Design review of the part built by this model. Coordinates are the model's own, in mm. Face numbers are marked on the shaded views. Coordinates: 2 decimals unless noted, no trailing zeros. Write each loop counter-clockwise with the first axis right and the second up, starting at its lowest first coordinate (ties: lowest second). Pieces come first, ordered by that corner, then holes. Notation, with made-up numbers: (10, 49) -> (62, 49) arc R29 cw to (62, 86) -> close; hole circle Ø9 at (87, 63.5). An arc over 180 degrees is marked (long way). Write item = value, one per line. Start each with the question number.
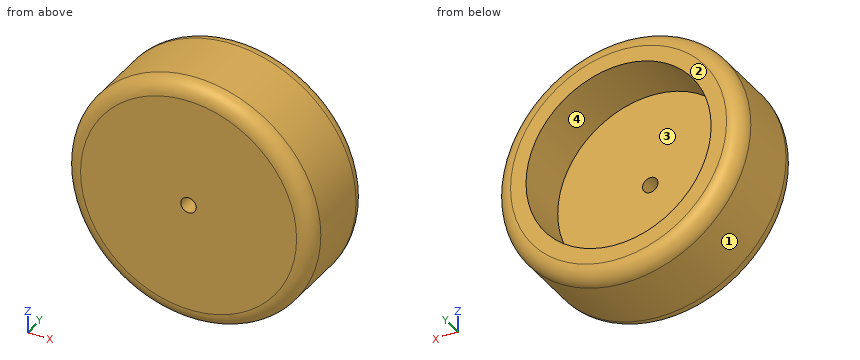
```python
from build123d import *

# Parameters (mm, degrees)
F0_R     = 40
F1_DEPTH = 30
F2_R     = 5
F3_R     = 30
F4_DEPTH = 18
F5_R     = 2.5
F6_DEPTH = 41.9


with BuildPart() as f1:
    # F0 (on Front) → F1 (new body)
    with BuildSketch(Plane.XZ):
        Circle(F0_R)
    extrude(amount=F1_DEPTH)

    # F2
    f2_edges = [f1.edges().sort_by_distance(p)[0] for p in [
        (40, -15, 0),
        (-40, 0, 0),
        (-40, -30, 0),
    ]]
    fillet(f2_edges, radius=F2_R)

    # F3 (on Front) → F4 (cut)
    with BuildSketch(Plane.XZ):
        Circle(F3_R)
    extrude(amount=F4_DEPTH, mode=Mode.SUBTRACT)

    # F5 (on Front) → F6 (cut)
    with BuildSketch(Plane.XZ):
        Circle(F5_R)
    extrude(amount=F6_DEPTH, mode=Mode.SUBTRACT)


solid = f1.part
```
(1) Mouldability with a two-part tool opening along Z and no side actions: class the marked faces 1, 2, 3 and 4 as pulls with the +Z half, pulls with the -Z half, needs draft (parallel to the pull), parting line crosses it, or undercut.
(2) For line 1 (Z direction, x = 0, y = -23.5); line 2 (Z direction, x = 0, y = -9.5); line 3 (X direction, y = -16, z = -1), list the stretches that pass through material, from the lowest coordinate up.
(3) Take a section at C-C, the plane y = -11. State the section outline as (x, z) points.
(4) Take a section at A-A, the plane z = 0. State the section outline as (x, y) points.
(5) For pin 1 Ø2 at (y, z) = (-12, -26) entering from +X (3 decimals); pin 2 Ø6.5 at (x, z) = (0, 0) entering from -Y; pin 3 Ø3 at (x, y) = (29, -19.5) entering from -Z; pin 4 Ø4 at (x, z) = (10.5, 12.5) entering from +Y, all flat-tipped, find the tip position at first contact; note any pin that passes through.
(6) Take a section at B-B, the plane x = 0. State the section outline as (y, z) points, then the cut area to 3 significant figures.
(7) Take a section at D-D, the plane y = -22. State the section outline as (x, z) points.
Report:
q1.face_1 = parting line crosses it
q1.face_2 = needs draft
q1.face_3 = undercut
q1.face_4 = undercut
q2.line_1 = -40 to -2.5, 2.5 to 40
q2.line_2 = -40 to -30, 30 to 40
q2.line_3 = -39.99 to -29.98, 29.98 to 39.99
q3.outline = circle Ø80 at (0, 0); hole circle Ø60 at (0, 0)
q4.outline = (-40, -25) arc R5 ccw to (-35, -30) -> (-2.5, -30) -> (-2.5, -18) -> (-30, -18) -> (-30, 0) -> (-35, 0) arc R5 ccw to (-40, -5) -> close; (2.5, -30) -> (35, -30) arc R5 ccw to (40, -25) -> (40, -5) arc R5 ccw to (35, 0) -> (30, 0) -> (30, -18) -> (2.5, -18) -> close
q5.pin_1 = 31.225
q5.pin_2 = -30
q5.pin_3 = -29.05
q5.pin_4 = -18
q6.outline = (-30, -35) arc R5 ccw to (-25, -40) -> (-5, -40) arc R5 ccw to (0, -35) -> (0, -30) -> (-18, -30) -> (-18, -2.5) -> (-30, -2.5) -> close; (-30, 2.5) -> (-18, 2.5) -> (-18, 30) -> (0, 30) -> (0, 35) arc R5 ccw to (-5, 40) -> (-25, 40) arc R5 ccw to (-30, 35) -> close
q6.area = 1,240 mm2
q7.outline = circle Ø80 at (0, 0); hole circle Ø5 at (0, 0)
